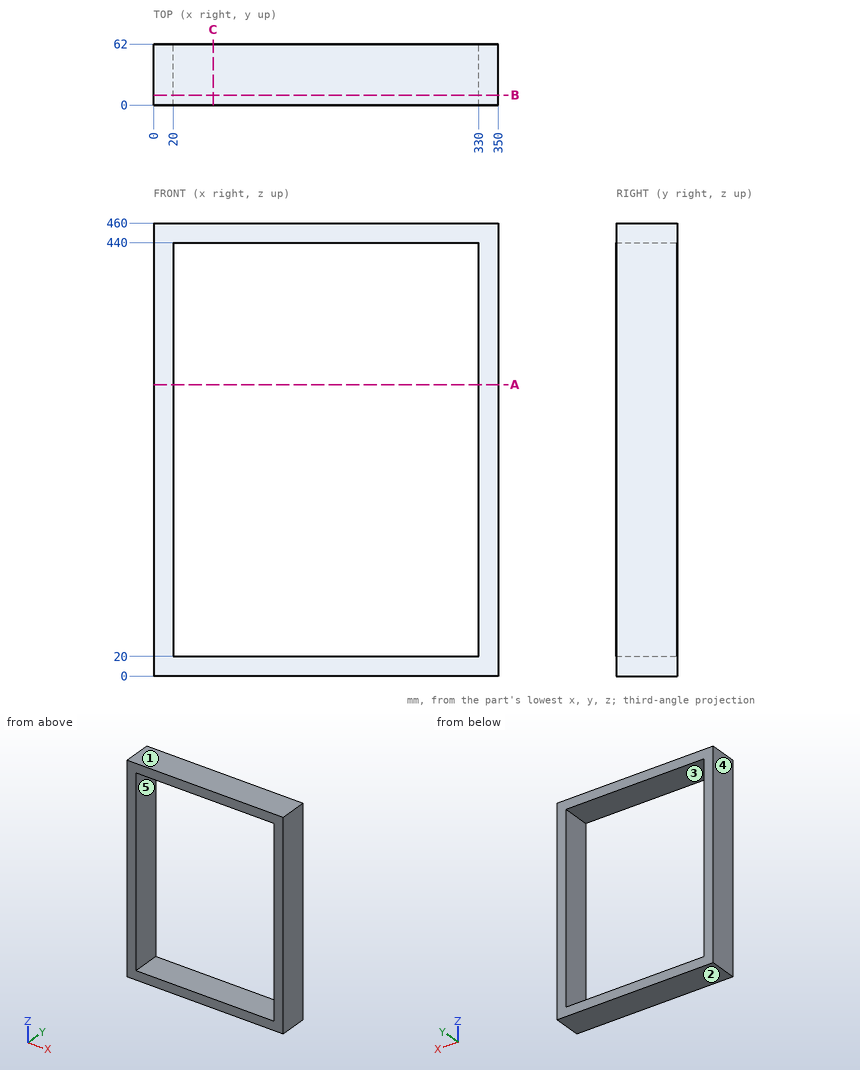
Print and shaded views of the part. All mm, measured from the part's lowest x, y and z. A direction names the side the tool comes from. Round coordinates to 2 decimals unless told otherwise and drop trailing zeros. Loops run counter-clockwise (first coordinate to the right, second up) from the corner with the lowest first, then second, coordinate; pieces in that order, holes last. Notation, with made-up numbers: M 1,80 L 19,80 A14 cw 19,93 Z; hole C 55,23.5 d9. An arc over 180 degrees is marked long. One line per question, with ' | ' between items.
1) Mould opens along Z. For the marked faces 1, 2 and 3 say: +Z half, -Z half, draft (parallel to the pull), parting line (faces both ways), or undercut.
Solved:
face 1: +Z half | face 2: -Z half | face 3: undercut
2) Band-saw the part on C-C (x = 60.5). Give the cut face in (y, z), then the cut area to 3 significant figures.
Solved:
outline: M 0,0 L 62,0 L 62,20 L 0,20 Z; M 0,440 L 62,440 L 62,460 L 0,460 Z | area: 2,480 mm²
3) 3-axis set-ups, long thin cutter, end or side, ignore diameter. For the marked faces 4 and 5: which of +Z, -Z, +X, -X, +Y, -Y reach the whole face in a straight line?
Solved:
face 4: +Z, -Z, -X, +Y, -Y | face 5: +Y, -Y
4) Band-saw the part on A-A (z = 296). Give the cut face in (x, y).
Solved:
outline: M 0,0 L 20,0 L 20,62 L 0,62 Z; M 330,0 L 350,0 L 350,62 L 330,62 Z
5) Band-saw the part on B-B (y = 10). Give the cut face in (x, z), then the cut area to 3 significant figures.
Solved:
outline: M 0,0 L 350,0 L 350,460 L 0,460 Z; hole M 20,20 L 330,20 L 330,440 L 20,440 Z | area: 30,800 mm²
6) Drill centre lines: line 1 along X through (y, z) = (12.5, 72); line 2 along Z through (x, y) = (216.5, 10). Where is each one in solid material? Low to high.
Solved:
line 1: x = 0 to 20, 330 to 350 | line 2: z = 0 to 20, 440 to 460
